```python
from build123d import *

# Parameters (mm, degrees)
EXTRUDE_1_DEPTH     = 3
SKETCH_2_R          = 1.5
CUT_EXTRUDE_1_DEPTH = 3


with BuildPart() as part:
    # 草图1 → 凸台-拉伸1 (new body)
    with BuildSketch(Plane.XY):
        with BuildLine():
            Line((-7.5, 0), (7.5, 0))
            Line((7.5, 0), (25, -23))
            Line((25, -23), (25, -38))
            Line((25, -38), (-25, -38))
            Line((-25, -38), (-57.5, -38))
            Line((-57.5, -38), (-57.5, 7))
            Line((-57.5, 7), (-42.5, 7))
            Line((-42.5, 7), (-42.5, -13))
            ThreePointArc((-42.5, -13), (-39.571067812, -20.071067812), (-32.5, -23))
            Line((-32.5, -23), (-29.956822623, -23))
            ThreePointArc((-29.956822623, -23), (-25.515661922, -21.959692608), (-21.998535682, -19.055218325))
            Line((-21.998535682, -19.055218325), (-7.5, 0))
        make_face()
    extrude(amount=EXTRUDE_1_DEPTH)

    # 草图2 → 切除-拉伸1 (cut)
    with BuildSketch(Plane.XY.offset(3)):
        with Locations((0, -4)):
            Circle(SKETCH_2_R)
        with Locations((0, -17)):
            Circle(SKETCH_2_R)
        with Locations((-21, -30.5)):
            Circle(SKETCH_2_R)
        with Locations((21, -30.5)):
            Circle(SKETCH_2_R)
        with Locations((-50, 0)):
            Circle(SKETCH_2_R)
        with Locations((-50, -18)):
            Circle(SKETCH_2_R)
    extrude(amount=-CUT_EXTRUDE_1_DEPTH, mode=Mode.SUBTRACT)


solid = part.part
```
Work out the finished part from the listing and answer in its coordinate system (mm). A direction names the side the tool comes from. Coordinates: 2 decimals unless noted, no trailing zeros. Loops run counter-clockwise (first coordinate to the right, second up) from the corner with the lowest first, then second, coordinate; pieces in that order, holes last.
1) For faces 4 (the flat face through (-50, 7, 1)), 5 (the flat face through (-42.5, -3, 1)), 6 (the flat face through (0, 0, 1)), determine the directions among +Z, -Z, +X, -X, +Y, -Y from which every point of the face is accessible in a straight line to the end or side of a thin tool.
Results:
face 4: +Z, -Z, +X, -X, +Y
face 5: +Z, -Z, +Y
face 6: +Z, -Z, +X, +Y
2) Section C-C (z = 1.7) is taken. Give the vertices of the cut face in (x, y).
Results:
outline: (-57.5, -38) - (25, -38) - (25, -23) - (7.5, 0) - (-7.5, 0) - (-22, -19.06) arc R10 cw to (-29.96, -23) - (-32.5, -23) arc R10 cw to (-42.5, -13) - (-42.5, 7) - (-57.5, 7) - close; hole circle Ø3 at (-50, -18); hole circle Ø3 at (-50, 0); hole circle Ø3 at (-21, -30.5); hole circle Ø3 at (0, -17); hole circle Ø3 at (0, -4); hole circle Ø3 at (21, -30.5)
3) Section B-B (x = -50) is taken. Give the vertices of the cut face in (y, z), plus the area to 3 significant figures.
Results:
outline: (-38, 0) - (-19.5, 0) - (-19.5, 3) - (-38, 3) - close; (-16.5, 0) - (-1.5, 0) - (-1.5, 3) - (-16.5, 3) - close; (1.5, 0) - (7, 0) - (7, 3) - (1.5, 3) - close
area: 117 mm2
4) Section D-D (y = -7.5) is taken. Give the vertices of the cut face in (x, z), plus the area to 3 significant figures.
Results:
outline: (-57.5, 0) - (-42.5, 0) - (-42.5, 3) - (-57.5, 3) - close; (-13.21, 0) - (13.21, 0) - (13.21, 3) - (-13.21, 3) - close
area: 124 mm2
5) Consider probe 1 along Y at (x, z) = (0, 2.3); probe 2 along X at (y, z) = (-16, 0.9); probe 3 along Y at (x, z) = (-49, 0.1). Determine where each line is inside the solid, lowest interval first.
Results:
probe 1: y = -38 to -18.5, -15.5 to -5.5, -2.5 to 0
probe 2: x = -57.5 to -42.04, -19.67 to -1.12, 1.12 to 19.67
probe 3: y = -38 to -19.12, -16.88 to -1.12, 1.12 to 7
6) Flat-ended cylindrical pins translate along their axes: pin 1 (3 mm diameter, centred on x = -11, y = -15.5, fed in from -Z); pin 2 (1.5 mm diameter, centred on x = -6.5, z = 2.5, fed in from +Y); pin 3 (1.5 mm diameter, centred on y = -5.5, z = 2, fed in from +X). Find the tip coordinate at first contact, or state that the pin passes through.
Results:
pin 1: stops at z = 0
pin 2: stops at y = 0
pin 3: stops at x = 12.26
7) For a pull along Y with two mould halves and no side action, classify faces 1 (the cylindrical face through (-25.6, -22, 1.5)), 2 (the flat face through (-57.5, -16, 1)), 3 (the cylindrical face through (-0.195, -15.513, 1.521)) as +Y half, -Y half, draft (parallel to the pull), parting line (faces both ways), or undercut.
Results:
face 1: +Y half
face 2: draft
face 3: undercut
8) Section A-A (y = -30.5) is taken. Give the vertices of the cut face in (x, z), plus the area to 4 significant figures.
Results:
outline: (-57.5, 0) - (-22.5, 0) - (-22.5, 3) - (-57.5, 3) - close; (-19.5, 0) - (19.5, 0) - (19.5, 3) - (-19.5, 3) - close; (22.5, 0) - (25, 0) - (25, 3) - (22.5, 3) - close
area: 229.5 mm2
